Here's how the part is built. I have some questions about the finished solid (model axes, mm). Face numbers are marked on the shaded views. A direction names the side the tool comes from. Give positions to 0.01 mm unless a question says otherwise; leave off trailing zeros. Loops run counter-clockwise (first coordinate to the right, second up) from the corner with the lowest first, then second, coordinate; pieces in that order, holes last.
Q1. We'd pull the mould along Y, two halves only. Please class the marked faces 1, 2, 3 and 4: +Y half, -Y half, draft (parallel to the pull), parting line (faces both ways), or undercut.
Q2. If we section it at A-A (z = 3.45): Please give me the cut outline in (x, y), plus the area to 3 significant figures.
Q3. Will these pins go through, and if not, where does the flat tip stop? P1, Ø1.2, axis at y = -11.5, z = 2.5, coming from the -X side; P2, Ø2, axis at x = 0.5, z = 4, coming from the +Y side; P3, Ø1.6, axis at x = -2.5, y = -12, coming from the +Z side.
Q4. If we section it at B-B (y = 0): Please give me the cut outline in (x, z).
Q5. I need wall thicknesses on line 1 (Z direction, x = 2, y = -8.75); line 2 (Z direction, x = 1, y = -5.25); line 3 (X direction, y = -11.25, z = 2.55). Which ranges of each line are inside material? Lowest first, please.
Q6. If we section it at C-C (x = 0): Please give me the cut outline in (y, z).
Q7. If we section it at D-D (y = -11.75): Please give me the cut outline in (x, z).
Q8. For the marked faces 5, 6, 7 and 8, which set-ups out of +Z, -Z, +X, -X, +Y, -Y let a thin tool reach every point of the face, with its end or its side?
from build123d import *

# Parameters (mm, degrees)
EXTRUDE_1_DEPTH = 1
SKETCH_2_R      = 4.5
EXTRUDE_2_DEPTH = 5
SKETCH_3_W      = 11.148375858
SKETCH_3_H      = 5.169406936
EXTRUDE_3_DEPTH = 4


with BuildPart() as part:
    # 草图1 → 凸台-拉伸1 (new body)
    with BuildSketch(Plane.XY):
        with BuildLine():
            Line((-2.275007411, 5), (2.275007411, 5))
            ThreePointArc((2.275007411, 5), (4.76799478, 3.967370821), (5.800623959, 1.474383452))
            Line((5.800623959, 1.474383452), (5.800623959, -13))
            Line((5.800623959, -13), (-5.800623959, -13))
            Line((-5.800623959, -13), (-5.800623959, 1.474383452))
            ThreePointArc((-5.800623959, 1.474383452), (-4.76799478, 3.967370821), (-2.275007411, 5))
        make_face()
    extrude(amount=EXTRUDE_1_DEPTH)

    # 草图2 → 凸台-拉伸2 (add)
    with BuildSketch(Plane.XY.offset(1)):
        Circle(SKETCH_2_R)
    extrude(amount=EXTRUDE_2_DEPTH)

    # 草图3 → 凸台-拉伸3 (add)
    with BuildSketch(Plane.XY.offset(1)):
        with Locations((0, -10.837924987)):
            Rectangle(SKETCH_3_W, SKETCH_3_H)
    extrude(amount=EXTRUDE_3_DEPTH)


solid = part.part
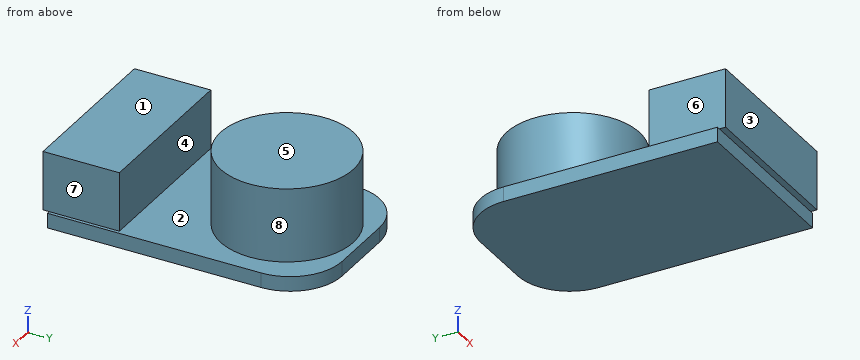
Check sheet entries:
1. face 1: draft
1. face 2: undercut
1. face 3: -Y half
1. face 4: undercut
2. outline: (-5.57, -13.42) - (5.57, -13.42) - (5.57, -8.25) - (-5.57, -8.25) - close; circle Ø9 at (0, 0)
2. area: 121 mm2
3. P1: stops at x = -5.57
3. P2: stops at y = 4.5
3. P3: stops at z = 5
4. outline: (-5.8, 0) - (5.8, 0) - (5.8, 1) - (4.5, 1) - (4.5, 6) - (-4.5, 6) - (-4.5, 1) - (-5.8, 1) - close
5. line 1: z = 0 to 5
5. line 2: z = 0 to 1
5. line 3: x = -5.57 to 5.57
6. outline: (-13.42, 1) - (-13, 1) - (-13, 0) - (5, 0) - (5, 1) - (4.5, 1) - (4.5, 6) - (-4.5, 6) - (-4.5, 1) - (-8.25, 1) - (-8.25, 5) - (-13.42, 5) - close
7. outline: (-5.8, 0) - (5.8, 0) - (5.8, 1) - (5.57, 1) - (5.57, 5) - (-5.57, 5) - (-5.57, 1) - (-5.8, 1) - close
8. face 5: +Z, +X, -X, +Y, -Y
8. face 6: +Z, -X, +Y, -Y
8. face 7: +Z, +X, +Y, -Y
8. face 8: +Z
